from build123d import *

# Parameters (mm, degrees)
SKETCH1_W                = 355.6
SKETCH1_H                = 76.2
BOSS_EXTRUDE1_DEPTH      = 6.35
SKETCH2_W                = 12.7
SKETCH2_H                = 25.4
CUT_EXTRUDE5_DEPTH       = 182.94716953
LPATTERN1_COUNT          = 13
LPATTERN1_PITCH          = 25.4
MIRROR1_COPY_1_SKETCH_W  = 12.7
MIRROR1_COPY_1_SKETCH_H  = 25.4
MIRROR1_COPY_1_DEPTH     = 182.94716953
MIRROR1_COPY_2_SKETCH_W  = 12.7
MIRROR1_COPY_2_SKETCH_H  = 25.4
MIRROR1_COPY_2_DEPTH     = 182.94716953
MIRROR1_COPY_3_SKETCH_W  = 12.7
MIRROR1_COPY_3_SKETCH_H  = 25.4
MIRROR1_COPY_3_DEPTH     = 182.94716953
MIRROR1_COPY_4_SKETCH_W  = 12.7
MIRROR1_COPY_4_SKETCH_H  = 25.4
MIRROR1_COPY_4_DEPTH     = 182.94716953
MIRROR1_COPY_5_SKETCH_W  = 12.7
MIRROR1_COPY_5_SKETCH_H  = 25.4
MIRROR1_COPY_5_DEPTH     = 182.94716953
MIRROR1_COPY_6_SKETCH_W  = 12.7
MIRROR1_COPY_6_SKETCH_H  = 25.4
MIRROR1_COPY_6_DEPTH     = 182.94716953
MIRROR1_COPY_7_SKETCH_W  = 12.7
MIRROR1_COPY_7_SKETCH_H  = 25.4
MIRROR1_COPY_7_DEPTH     = 182.94716953
MIRROR1_COPY_8_SKETCH_W  = 12.7
MIRROR1_COPY_8_SKETCH_H  = 25.4
MIRROR1_COPY_8_DEPTH     = 182.94716953
MIRROR1_COPY_9_SKETCH_W  = 12.7
MIRROR1_COPY_9_SKETCH_H  = 25.4
MIRROR1_COPY_9_DEPTH     = 182.94716953
MIRROR1_COPY_10_SKETCH_W = 12.7
MIRROR1_COPY_10_SKETCH_H = 25.4
MIRROR1_COPY_10_DEPTH    = 182.94716953
MIRROR1_COPY_11_SKETCH_W = 12.7
MIRROR1_COPY_11_SKETCH_H = 25.4
MIRROR1_COPY_11_DEPTH    = 182.94716953
MIRROR1_COPY_12_SKETCH_W = 12.7
MIRROR1_COPY_12_SKETCH_H = 25.4
MIRROR1_COPY_12_DEPTH    = 182.94716953
SKETCH3_W                = 40.748476415
SKETCH3_H                = 6.35
SKETCH3_W_2              = 25.4
SKETCH3_H_2              = 25.4
CUT_EXTRUDE7_DEPTH       = 182.94716953


with BuildPart() as part:
    # Sketch1 → Boss-Extrude1 (new body)
    with BuildSketch(Plane.XY):
        Rectangle(SKETCH1_W, SKETCH1_H)
    extrude(amount=BOSS_EXTRUDE1_DEPTH)

    # Sketch2 → Cut-Extrude5 (cut, symmetric)
    with BuildSketch(Plane.XY):
        with Locations((152.4, -44.45)):
            Rectangle(SKETCH2_W, SKETCH2_H)
    cut_extrude5 = extrude(amount=CUT_EXTRUDE5_DEPTH, both=True, mode=Mode.SUBTRACT)

    # LPattern1: Cut-Extrude5 ×13
    with Locations(*[(-i * LPATTERN1_PITCH, 0, 0) for i in range(1, LPATTERN1_COUNT)]):
        add(cut_extrude5, mode=Mode.SUBTRACT)

    # Mirror1: Cut-Extrude5 across plane
    add(cut_extrude5.mirror(Plane.ZX), mode=Mode.SUBTRACT)

    # Mirror1 copy 1 sketch → Mirror1 copy 1 (cut, symmetric)
    with BuildSketch(Plane(origin=(-25.4, 0, 0), x_dir=(1, 0, 0), z_dir=(0, 0, 1))):
        with Locations((152.4, 44.45)):
            Rectangle(MIRROR1_COPY_1_SKETCH_W, MIRROR1_COPY_1_SKETCH_H)
    extrude(amount=MIRROR1_COPY_1_DEPTH, both=True, mode=Mode.SUBTRACT)

    # Mirror1 copy 2 sketch → Mirror1 copy 2 (cut, symmetric)
    with BuildSketch(Plane(origin=(-50.8, 0, 0), x_dir=(1, 0, 0), z_dir=(0, 0, 1))):
        with Locations((152.4, 44.45)):
            Rectangle(MIRROR1_COPY_2_SKETCH_W, MIRROR1_COPY_2_SKETCH_H)
    extrude(amount=MIRROR1_COPY_2_DEPTH, both=True, mode=Mode.SUBTRACT)

    # Mirror1 copy 3 sketch → Mirror1 copy 3 (cut, symmetric)
    with BuildSketch(Plane(origin=(-76.2, 0, 0), x_dir=(1, 0, 0), z_dir=(0, 0, 1))):
        with Locations((152.4, 44.45)):
            Rectangle(MIRROR1_COPY_3_SKETCH_W, MIRROR1_COPY_3_SKETCH_H)
    extrude(amount=MIRROR1_COPY_3_DEPTH, both=True, mode=Mode.SUBTRACT)

    # Mirror1 copy 4 sketch → Mirror1 copy 4 (cut, symmetric)
    with BuildSketch(Plane(origin=(-101.6, 0, 0), x_dir=(1, 0, 0), z_dir=(0, 0, 1))):
        with Locations((152.4, 44.45)):
            Rectangle(MIRROR1_COPY_4_SKETCH_W, MIRROR1_COPY_4_SKETCH_H)
    extrude(amount=MIRROR1_COPY_4_DEPTH, both=True, mode=Mode.SUBTRACT)

    # Mirror1 copy 5 sketch → Mirror1 copy 5 (cut, symmetric)
    with BuildSketch(Plane(origin=(-127, 0, 0), x_dir=(1, 0, 0), z_dir=(0, 0, 1))):
        with Locations((152.4, 44.45)):
            Rectangle(MIRROR1_COPY_5_SKETCH_W, MIRROR1_COPY_5_SKETCH_H)
    extrude(amount=MIRROR1_COPY_5_DEPTH, both=True, mode=Mode.SUBTRACT)

    # Mirror1 copy 6 sketch → Mirror1 copy 6 (cut, symmetric)
    with BuildSketch(Plane(origin=(-152.4, 0, 0), x_dir=(1, 0, 0), z_dir=(0, 0, 1))):
        with Locations((152.4, 44.45)):
            Rectangle(MIRROR1_COPY_6_SKETCH_W, MIRROR1_COPY_6_SKETCH_H)
    extrude(amount=MIRROR1_COPY_6_DEPTH, both=True, mode=Mode.SUBTRACT)

    # Mirror1 copy 7 sketch → Mirror1 copy 7 (cut, symmetric)
    with BuildSketch(Plane(origin=(-177.8, 0, 0), x_dir=(1, 0, 0), z_dir=(0, 0, 1))):
        with Locations((152.4, 44.45)):
            Rectangle(MIRROR1_COPY_7_SKETCH_W, MIRROR1_COPY_7_SKETCH_H)
    extrude(amount=MIRROR1_COPY_7_DEPTH, both=True, mode=Mode.SUBTRACT)

    # Mirror1 copy 8 sketch → Mirror1 copy 8 (cut, symmetric)
    with BuildSketch(Plane(origin=(-203.2, 0, 0), x_dir=(1, 0, 0), z_dir=(0, 0, 1))):
        with Locations((152.4, 44.45)):
            Rectangle(MIRROR1_COPY_8_SKETCH_W, MIRROR1_COPY_8_SKETCH_H)
    extrude(amount=MIRROR1_COPY_8_DEPTH, both=True, mode=Mode.SUBTRACT)

    # Mirror1 copy 9 sketch → Mirror1 copy 9 (cut, symmetric)
    with BuildSketch(Plane(origin=(-228.6, 0, 0), x_dir=(1, 0, 0), z_dir=(0, 0, 1))):
        with Locations((152.4, 44.45)):
            Rectangle(MIRROR1_COPY_9_SKETCH_W, MIRROR1_COPY_9_SKETCH_H)
    extrude(amount=MIRROR1_COPY_9_DEPTH, both=True, mode=Mode.SUBTRACT)

    # Mirror1 copy 10 sketch → Mirror1 copy 10 (cut, symmetric)
    with BuildSketch(Plane(origin=(-254, 0, 0), x_dir=(1, 0, 0), z_dir=(0, 0, 1))):
        with Locations((152.4, 44.45)):
            Rectangle(MIRROR1_COPY_10_SKETCH_W, MIRROR1_COPY_10_SKETCH_H)
    extrude(amount=MIRROR1_COPY_10_DEPTH, both=True, mode=Mode.SUBTRACT)

    # Mirror1 copy 11 sketch → Mirror1 copy 11 (cut, symmetric)
    with BuildSketch(Plane(origin=(-279.4, 0, 0), x_dir=(1, 0, 0), z_dir=(0, 0, 1))):
        with Locations((152.4, 44.45)):
            Rectangle(MIRROR1_COPY_11_SKETCH_W, MIRROR1_COPY_11_SKETCH_H)
    extrude(amount=MIRROR1_COPY_11_DEPTH, both=True, mode=Mode.SUBTRACT)

    # Mirror1 copy 12 sketch → Mirror1 copy 12 (cut, symmetric)
    with BuildSketch(Plane(origin=(-304.8, 0, 0), x_dir=(1, 0, 0), z_dir=(0, 0, 1))):
        with Locations((152.4, 44.45)):
            Rectangle(MIRROR1_COPY_12_SKETCH_W, MIRROR1_COPY_12_SKETCH_H)
    extrude(amount=MIRROR1_COPY_12_DEPTH, both=True, mode=Mode.SUBTRACT)

    # Sketch3 → Cut-Extrude7 (cut, through all)
    with BuildSketch(Plane.XY):
        with Locations((191.824238208, 19.05)):
            Rectangle(SKETCH3_W, SKETCH3_H)
        with Locations((191.824238208, 6.35)):
            Rectangle(SKETCH3_W, SKETCH3_H)
        with Locations((191.824238208, -6.35)):
            Rectangle(SKETCH3_W, SKETCH3_H)
        with Locations((191.824238208, -19.05)):
            Rectangle(SKETCH3_W, SKETCH3_H)
        with Locations((184.15, 44.45)):
            Rectangle(SKETCH3_W_2, SKETCH3_H_2)
        with Locations((184.15, -44.45)):
            Rectangle(SKETCH3_W_2, SKETCH3_H_2)
    cut_extrude7 = extrude(amount=CUT_EXTRUDE7_DEPTH, mode=Mode.SUBTRACT)

    # Mirror2: Cut-Extrude7 across plane
    add(cut_extrude7.mirror(Plane(origin=(0, 0, 0), x_dir=(0, 0, 1), z_dir=(1, 0, 0))), mode=Mode.SUBTRACT)


solid = part.part
The listing builds one solid part. Answer for the finished solid, in the listing's coordinates (mm). A direction names the side the tool comes from. Round coordinates to 2 decimals unless told otherwise and drop trailing zeros. Order: outer loops, then holes, each group sorted by start corner. A loop starts at its lowest first (then second) coordinate and runs counter-clockwise, first axis right, second up. Notation, with made-up numbers: (71, -1) -> (107, -1) arc R25 ccw to (107, 28) -> close; hole circle Ø5 at (85.5, 76). An arc over 180 degrees is marked (long way). One line per item, written item: value.
Item 1: For faces 5 (the flat face through (-64, 38.1, 3)), 6 (the flat face through (127, 31.75, 3)), 7 (the flat face through (107.95, -35, 3)), 8 (the flat face through (171.45, -19, 3)), determine the directions among +Z, -Z, +X, -X, +Y, -Y from which every point of the face is accessible in a straight line to the end or side of a thin tool.
Taken from the geometry:
face 5: +Z, -Z, +X, -X, +Y
face 6: +Z, -Z, +Y
face 7: +Z, -Z, -Y
face 8: +Z, -Z, +X
Item 2: Find section A-A, the plane x = -124. Give the vertices of the cut face in (y, z).
Taken from the geometry:
outline: (-31.75, 0) -> (31.75, 0) -> (31.75, 6.35) -> (-31.75, 6.35) -> close
Item 3: For a pull along X with two mould halves and no side action, classify faces 1 (the flat face through (-57.15, -35, 3)), 2 (the flat face through (171.45, 19, 3)), 3 (the flat face through (-38, -38.1, 3)), 4 (the flat face through (-171.45, -6, 3)) as released by +X, released by -X, zero draft, split by the parting line, or undercut.
Taken from the geometry:
face 1: undercut
face 2: released by +X
face 3: zero draft
face 4: released by -X
Item 4: Straight lines are drawn through the part: L1, parallel to Y at x = 148, z = 0.75; L2, parallel to X at y = 4.5, z = 2.25. For each, find the intervals that lie inside material, in ascending order.
Taken from the geometry:
L1: y = -31.75 to 31.75
L2: x = -171.45 to 171.45
Item 5: Given P1, Ø3, axis at y = -19, z = 4, coming from the +X side; P2, Ø3, axis at x = -126, z = 2, coming from the +Y side, each flat-ended and moving along its own axis, determine where each tip first touches the part or whether it passes through.
Taken from the geometry:
P1: stops at x = 171.45
P2: stops at y = 31.75
